Geometry: see drawing. Coordinates: mm, zero at the bounding-box minimum. Coordinates: 2 decimals unless noted, no trailing zeros. Put each result on its own line as item: value. Start each with the question number.
1) Cut plane B-B (x = 5.5). State how many separate pieces and enclosed holes the cut face has, plus the area to 3 significant figures.
2) Material intervals for L1, parallel to Z at x = 3, y = 8; L2, parallel to Z at x = 5.5, y = 6.25 (1 decimal); L3, parallel to Y at x = 4.5, z = 57.15 (1 decimal), sorted ascending.
3) Contact query for a flat-ended pin moving along its axis: P1, Ø4, axis at y = 7.94, z = 57.15, coming from the +X side. Output: stop coordinate, or through.
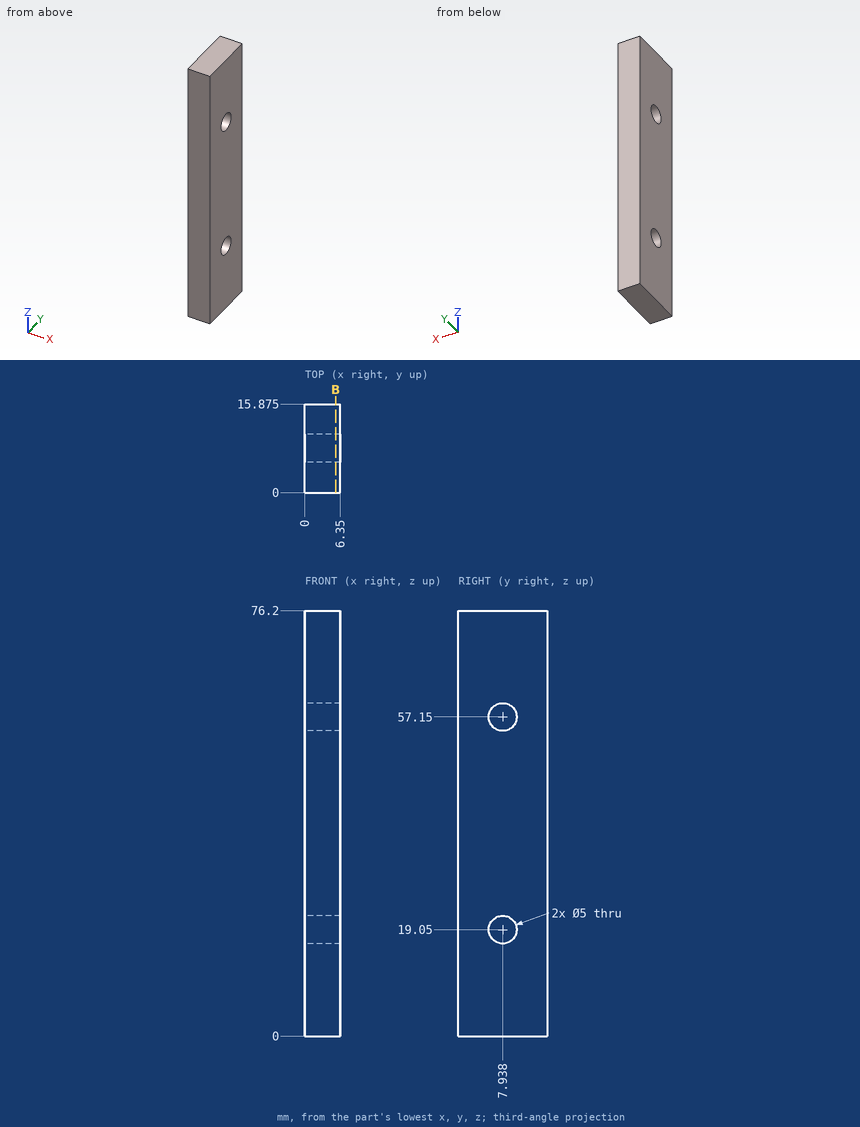
Results found:
1. separate pieces: 1
1. enclosed holes: 2
1. area: 1,170 mm2
2. L1: z = 0 to 16.55, 21.55 to 54.65, 59.65 to 76.2
2. L2: z = 0 to 17.2, 20.9 to 55.3, 59 to 76.2
2. L3: y = 0 to 5.4, 10.4 to 15.9
3. P1: passes through
